CAD build for the part. Positions are in the model's coordinates, mm. Round coordinates to 2 decimals unless told otherwise and drop trailing zeros. Write each loop counter-clockwise with the first axis right and the second up, starting at its lowest first coordinate (ties: lowest second). Pieces come first, ordered by that corner, then holes. Notation, with made-up numbers: (57.25, -38.75) -> (77.25, -38.75) arc R18 cw to (77.25, -28.75) -> close; hole circle Ø4 at (86, 44). An arc over 180 degrees is marked (long way). Answer in a Markdown table with one row per item. Add a question column.
```python
from build123d import *

# Parameters (mm, degrees)
BASENUTSKETCH_R = 10.5
BASENUT_DEPTH   = 21.5


with BuildPart() as part:
    # BaseNutSketch → BaseNut (new body)
    with BuildSketch(Plane(origin=(0, 0, 0), x_dir=(0, -1, 0), z_dir=(1, 0, 0))):
        Polygon((10.392304845, 18), (-10.392304845, 18), (-20.784609691, 0), (-10.392304845, -18), (10.392304845, -18), (20.784609691, 0), align=None)
        with Locations(Location((0, 0, 0), (0, 0, 90))):
            Circle(BASENUTSKETCH_R, mode=Mode.SUBTRACT)
    extrude(amount=BASENUT_DEPTH)


solid = part.part
```
Item 1: Saw through at C-C on z = 0.5. Give the cut face in (x, y), then the cut area to 3 significant figures.
Item 2: Drill centre lines: probe 1 along Y at (x, z) = (11.5, 0); probe 2 along Z at (x, y) = (2.5, 7); probe 3 along Y at (x, z) = (10.25, -9.5). Where is each one in solid material? Low to high.
Item 3: Pin check, flat tips, straight feed: pin 1 (1.5 mm diameter, centred on x = 2.5, z = 3, fed in from -Y); pin 2 (4 mm diameter, centred on x = 3.5, z = -7, fed in from +Y); pin 3 (1 mm diameter, centred on x = 14, z = -8.5, fed in from +Y); pin 4 (12 mm diameter, centred on x = 13, z = -4.5, fed in from -Y). Stop position of each tip, or through.
Item 4: Saw through at B-B on x = 3. Give the cut face in (y, z), then the cut area to 3 significant figures.
Item 5: Two-plate mould, pull along Y, no slides. Class faces 1 (the cylindrical face through (10.6, 3.2, -10)), 2 (the flat face through (10.599, -15.516, 9.126)), 3 (the flat face through (10.599, 15.516, -9.126)): +Y half, -Y half, draft (parallel to the pull), parting line (faces both ways), or undercut.
Item 6: Saw through at D-D on z = 12. Give the cut face in (x, y), then the cut area to 3 significant figures.
Item 7: Saw through at A-A on y = 0. Give the cut face in (x, z), then the cut area to 4 significant figures.
Recorded:
| question | item | result |
|---|---|---|
| 1 | outline | (0, -20.5) -> (21.5, -20.5) -> (21.5, -10.49) -> (0, -10.49) -> close; (0, 10.49) -> (21.5, 10.49) -> (21.5, 20.5) -> (0, 20.5) -> close |
| 1 | area | 430 mm2 |
| 2 | probe 1 | -20.78 to -10.5, 10.5 to 20.78 |
| 2 | probe 2 | -18 to -7.83, 7.83 to 18 |
| 2 | probe 3 | -15.3 to -4.47, 4.47 to 15.3 |
| 3 | pin 1 | y = -19.49 |
| 3 | pin 2 | y = 17.9 |
| 3 | pin 3 | y = 16.17 |
| 3 | pin 4 | y = -20.78 |
| 4 | outline | (-20.78, 0) -> (-10.39, -18) -> (10.39, -18) -> (20.78, 0) -> (10.39, 18) -> (-10.39, 18) -> close; hole circle Ø21 at (0, 0) |
| 4 | area | 776 mm2 |
| 5 | face 1 | undercut |
| 5 | face 2 | -Y half |
| 5 | face 3 | +Y half |
| 6 | outline | (0, -13.86) -> (21.5, -13.86) -> (21.5, 13.86) -> (0, 13.86) -> close |
| 6 | area | 596 mm2 |
| 7 | outline | (0, -18) -> (21.5, -18) -> (21.5, -10.5) -> (0, -10.5) -> close; (0, 10.5) -> (21.5, 10.5) -> (21.5, 18) -> (0, 18) -> close |
| 7 | area | 322.5 mm2 |
